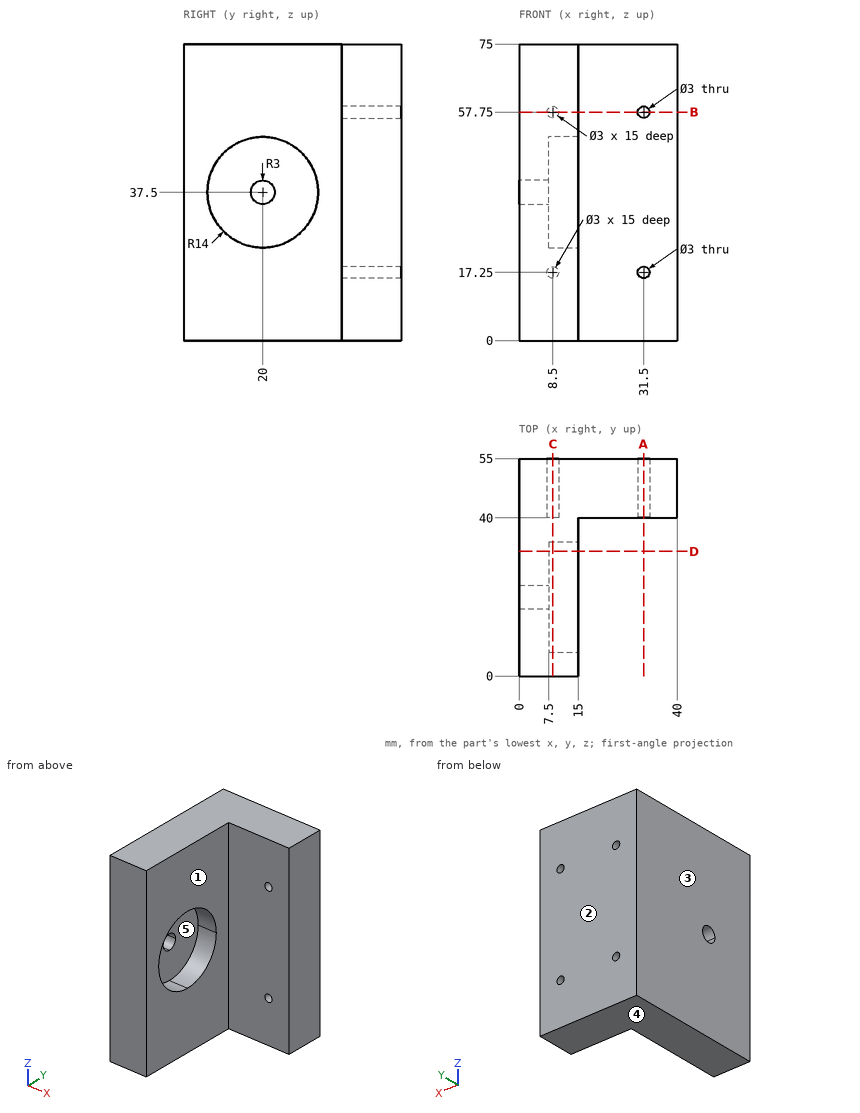
Can you work these out from the drawing? Everything is in mm from the part's minimum corner. A direction names the side the tool comes from. Give positions to 0.01 mm unless a question says otherwise; leave off trailing zeros. Order: outer loops, then holes, each group sorted by start corner. A loop starts at its lowest first (then second) coordinate and runs counter-clockwise, first axis right, second up. Notation, with made-up numbers: M 14.25,74.5 L 62.25,74.5 A20 cw 62.25,107.5 Z; hole C 5,25 d3. An arc over 180 degrees is marked long. Use a Markdown table: item, result. Add a question column.
1. If we mould it in two halves opening along Z, with no side actions, what happens to the marked faces 3, 4 and 5? For each: +Z half, -Z half, draft (parallel to the pull), parting line (faces both ways), or undercut.
2. For pin 1 Ø2.5 at (x, z) = (31.5, 17.25) entering from -Y; pin 2 Ø12.5 at (x, z) = (22.5, 19) entering from -Y; pin 3 Ø22.5 at (y, z) = (24, 43.5) entering from +X; pin 4 Ø1.5 at (x, z) = (8.5, 17.5) entering from +Y, each with a flat end and sliding along its axis, tell me the tip position at first contact or that it passes through.
3. On a 3-axis mill with a long thin cutter (end or side, diameter ignored), from which of +Z, -Z, +X, -X, +Y, -Y can I reach the whole of each face in a straight line? I mean the marked faces 1 and 2. Say none if no direction works.
4. I need wall thicknesses on probe 1 along X at (y, z) = (51.25, 17.25); probe 2 along X at (y, z) = (16.5, 30); probe 3 along Y at (x, z) = (20, 71). Which ranges of each line are inside material? Lowest first, please. Write a range as from..to.
5. Suppose I cut it at C-C (x = 8.5). List the corners of the cut face in (y, z) for me, and give its area (3 significant figures).
6. Suppose I cut it at A-A (x = 31.5). List the corners of the cut face in (y, z) for me, and give its area (4 significant figures).
7. Suppose I cut it at D-D (y = 31.5). List the corners of the cut face in (x, z) for me.
8. Suppose I cut it at B-B (z = 57.75). List the corners of the cut face in (x, y) for me, and give its area (3 significant figures).
Results list:
| question | item | result |
|---|---|---|
| 1 | face 3 | draft |
| 1 | face 4 | -Z half |
| 1 | face 5 | undercut |
| 2 | pin 1 | passes through |
| 2 | pin 2 | stops at y = 40 |
| 2 | pin 3 | stops at x = 15 |
| 2 | pin 4 | stops at y = 40 |
| 3 | face 1 | +Z, -Z, +X, -Y |
| 3 | face 2 | +Z, -Z, +X, -X, +Y |
| 4 | probe 1 | x = 0..7, 10..30, 33..40 |
| 4 | probe 2 | x = 0..7.5 |
| 4 | probe 3 | y = 40..55 |
| 5 | outline | M 0,0 L 55,0 L 55,15.75 L 40,15.75 L 40,18.75 L 55,18.75 L 55,56.25 L 40,56.25 L 40,59.25 L 55,59.25 L 55,75 L 0,75 Z; hole C 20,37.5 d28 |
| 5 | area | 3,420 mm² |
| 6 | outline | M 40,0 L 55,0 L 55,15.75 L 40,15.75 Z; M 40,18.75 L 55,18.75 L 55,56.25 L 40,56.25 Z; M 40,59.25 L 55,59.25 L 55,75 L 40,75 Z |
| 6 | area | 1,035 mm² |
| 7 | outline | M 0,0 L 15,0 L 15,29.52 L 7.5,29.52 L 7.5,45.48 L 15,45.48 L 15,75 L 0,75 Z |
| 8 | outline | M 0,0 L 15,0 L 15,40 L 30,40 L 30,55 L 10,55 L 10,40 L 7,40 L 7,55 L 0,55 Z; M 33,40 L 40,40 L 40,55 L 33,55 Z |
| 8 | area | 1,110 mm² |
